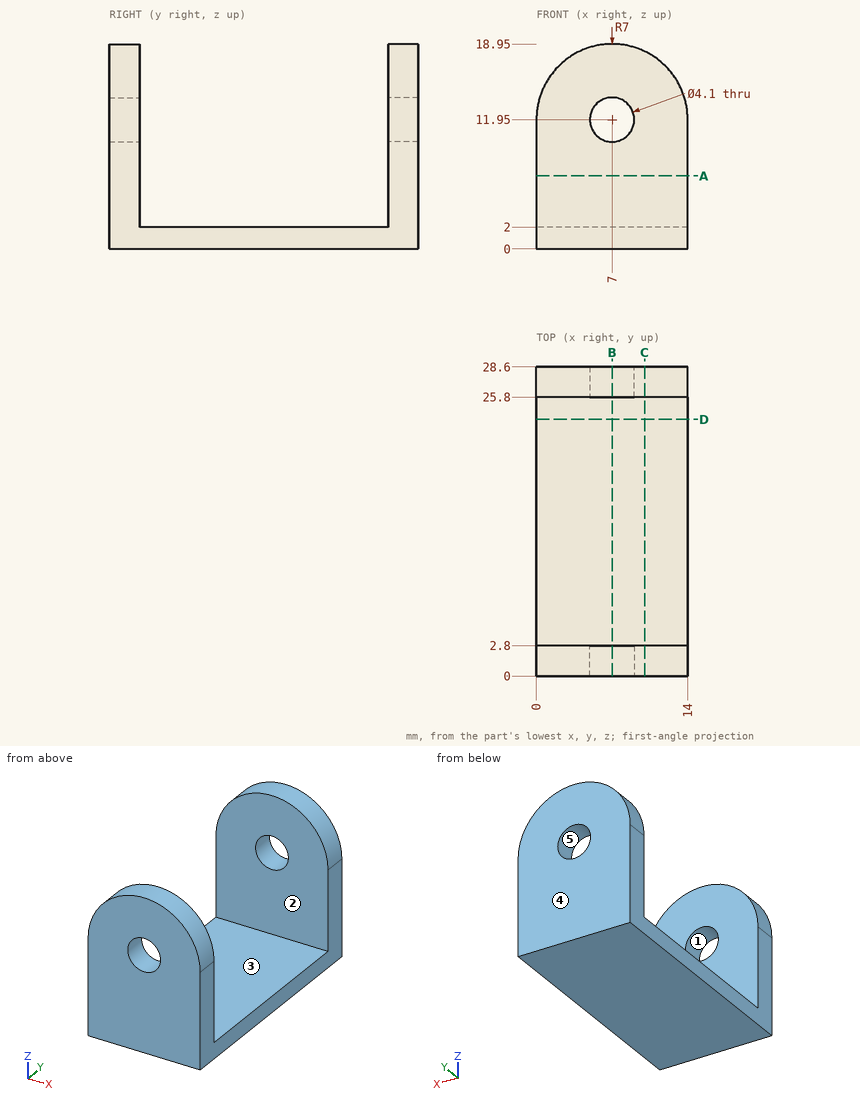
Source: three-view drawing plus pictorial views. Frame: mm from the lowest corner of the part. A direction names the side the tool comes from. Give positions to 0.01 mm unless a question says otherwise; leave off trailing zeros. Order: outer loops, then holes, each group sorted by start corner. A loop starts at its lowest first (then second) coordinate and runs counter-clockwise, first axis right, second up. Notation, with made-up numbers: (-33, -25.5) - (-14, -25.5) arc R7 cw to (-14, -21.5) - close; hole circle Ø3 at (34, 85.25). An arc over 180 degrees is marked (long way). Answer as a JSON object with one key per item and string values. Group by question number.
Q1. Mould query, pull axis Z, two halves, no side actions, for the marked faces 3, 4 and 5. Classes: pulls with the +Z half, pulls with the -Z half, needs draft (parallel to the pull), parting line crosses it, or undercut.
Q2. First-contact query: pin 1 Ø2.5 at (x, z) = (7, 11.95) entering from -Y. Flat tip, straight axial feed; report the tip coordinate or a pass-through.
Q3. Cut plane B-B, the plane x = 7. Output: boundary loops of the cut face in (y, z), then the cut area to 3 significant figures.
Q4. Set-up query: the marked faces 1 and 2. Return all of +Z, -Z, +X, -X, +Y, -Y with unobstructed straight access to the full face (end or side cutting, diameter ignored); none if empty.
Q5. Cut plane C-C, the plane x = 10. Output: boundary loops of the cut face in (y, z).
Q6. Line query: probe 1 along Z at (x, y) = (7, 27.2); probe 2 along Y at (x, z) = (6, 7.25); probe 3 along Z at (x, y) = (6.5, 19). Output: solid intervals per line, ascending.
Q7. Cut plane D-D, the plane y = 23.75. Output: boundary loops of the cut face in (x, z), then the cut area to 3 significant figures.
Q8. Cut plane A-A, the plane z = 6.75. Output: boundary loops of the cut face in (x, y), then the cut area to 3 significant figures.
Results:
{
 "1": {"face 3": "pulls with the +Z half", "face 4": "needs draft", "face 5": "undercut"},
 "2": {"pin 1": "through"},
 "3": {"outline": "(0, 0) - (28.6, 0) - (28.6, 9.9) - (25.8, 9.9) - (25.8, 2) - (2.8, 2) - (2.8, 9.9) - (0, 9.9) - close; (0, 14) - (2.8, 14) - (2.8, 18.95) - (0, 18.95) - close; (25.8, 14) - (28.6, 14) - (28.6, 18.95) - (25.8, 18.95) - close", "area": "129 mm^2"},
 "4": {"face 1": "+Y, -Y", "face 2": "+Z, +X, -X"},
 "5": {"outline": "(0, 0) - (28.6, 0) - (28.6, 18.27) - (25.8, 18.27) - (25.8, 2) - (2.8, 2) - (2.8, 18.27) - (0, 18.27) - close"},
 "6": {"probe 1": "0 to 9.9, 14 to 18.95", "probe 2": "0 to 2.8, 25.8 to 28.6", "probe 3": "0 to 2"},
 "7": {"outline": "(0, 0) - (14, 0) - (14, 2) - (0, 2) - close", "area": "28.0 mm^2"},
 "8": {"outline": "(0, 0) - (14, 0) - (14, 2.8) - (0, 2.8) - close; (0, 25.8) - (14, 25.8) - (14, 28.6) - (0, 28.6) - close", "area": "78.4 mm^2"}
}
